Autodesk Inventor part; units mm, degrees
ref_plane "YZ Plane" through (0, 0, 0) normal (1, 0, 0) x (0, 1, 0)
ref_plane "XZ Plane" through (0, 0, 0) normal (0, 1, 0) x (-1, 0, 0)
ref_plane "XY Plane" through (0, 0, 0) normal (0, 0, 1) x (1, 0, 0)
sketch "スケッチ1" plane through (0, 0, 0) normal (0, 0, 1) x (1, 0, 0)
  line L0 (9.4222, 72.3) -> (45.5, 72.3)
  arc A0 (50.5, 67.3) -> (45.5, 72.3) centre (45.5, 67.3) ccw
  line L1 (50.5, 67.3) -> (50.5, 43.9148)
  arc A1 (45.8359, 41.4187) -> (50.5, 43.9148) centre (47.5, 43.9148) ccw
  line L2 (45.8359, 41.4187) -> (7.7581, 66.8038)
  arc A2 (9.4222, 72.3) -> (7.7581, 66.8038) centre (9.4222, 69.3) ccw
  line L3 (31.5778, 32.3) -> (-4.5, 32.3)
  arc A3 (-9.5, 37.3) -> (-4.5, 32.3) centre (-4.5, 37.3) ccw
  line L4 (-9.5, 37.3) -> (-9.5, 60.6852)
  arc A4 (-4.8359, 63.1813) -> (-9.5, 60.6852) centre (-6.5, 60.6852) ccw
  line L5 (-4.8359, 63.1813) -> (33.2419, 37.7962)
  arc A5 (31.5778, 32.3) -> (33.2419, 37.7962) centre (31.5778, 35.3) ccw
  arc A6 (50.5, -32.7) -> (55.5, -27.7) centre (50.5, -27.7) ccw
  line L6 (55.5, -27.7) -> (55.5, 77.3)
  line L7 (55.5, 77.3) -> (-14.5, 77.3)
  line L8 (-14.5, 77.3) -> (-14.5, 27.3)
  line L9 (-14.5, 27.3) -> (-22.2876, 1.4419)
  arc A7 (-16.3774, 4.8724) -> (-22.2876, 1.4419) centre (-17.5, 0) ccw
  arc A8 (-16.3774, 4.8724) -> (-12.2872, 6.71) centre (-15.5442, 8.4886) ccw
  arc A9 (-7.5, 11.8216) -> (-12.2872, 6.71) centre (0, 0) ccw
  line L10 (-7.5, 11.8216) -> (-7.5, 18.5)
  arc A10 (-1.5, 24.5) -> (-7.5, 18.5) centre (-1.5, 18.5) ccw
  line L11 (-1.5, 24.5) -> (42.5, 24.5)
  arc A11 (48.5, 18.5) -> (42.5, 24.5) centre (42.5, 18.5) ccw
  line L12 (48.5, 18.5) -> (48.5, -8.5)
  line L13 (48.5, -8.5) -> (39.5, -8.5)
  arc A12 (31.5, -0.5) -> (39.5, -8.5) centre (39.5, -0.5) ccw
  line L14 (31.5, -0.5) -> (31.5, 8.5)
  line L15 (31.5, 8.5) -> (11.1243, 8.5)
  arc A13 (12.2844, 6.7152) -> (11.1243, 8.5) centre (0, 0) ccw
  arc A14 (12.2844, 6.7152) -> (16.3816, 4.8733) centre (15.5493, 8.5) ccw
  arc A15 (17.5, -5) -> (16.3816, 4.8733) centre (17.5, 0) ccw
  line L16 (17.5, -5) -> (10.0995, -5)
  arc A16 (8.3431, -3.9565) -> (10.0995, -5) centre (10.0995, -3) ccw
  arc A17 (8.3431, -3.9565) -> (-8.3431, -3.9565) centre (0, -8.5) ccw
  arc A18 (-10.0995, -5) -> (-8.3431, -3.9565) centre (-10.0995, -3) ccw
  line L17 (-10.0995, -5) -> (-17.5, -5)
  arc A19 (-22.5, 0) -> (-17.5, -5) centre (-17.5, 0) ccw
  line L18 (-22.5, 0) -> (-22.5, -27.7)
  arc A20 (-22.5, -27.7) -> (-17.5, -32.7) centre (-17.5, -27.7) ccw
  line L19 (-17.5, -32.7) -> (50.5, -32.7)
  circle A21 centre (-17.5, -27.7) radius 1.9
  circle A22 centre (50.5, -27.7) radius 1.9
  line L20 (55.5, -32.7) -> (-22.5, -32.7)
  line L21 (-22.5, -32.7) -> (-22.5, 5)
  line L22 (-22.5, 5) -> (55.5, 5)
  line L23 (55.5, 5) -> (55.5, -32.7)
  arc A23 (-16.3774, 4.8724) -> (-17.5, -5) centre (-17.5, 0) ccw
  point P0 (0, 0)
  point P1 (-17.5, 5)
extrude "押し出し1" add sketch "スケッチ1" along normal blind 3 contours L19 A20 L18 A19 L17 A18 A17 A16 L16 A15 L22 L14 A12 L13 L12 L6 A6 | L12 L13 A12 L14 L22 | A23 A7 A8 L22 A14 A15 L16 A16 A17 A18 L17 A19 | A15 A14 L22 | L22 A8 A7 | A21 | A22
fillet "フィレット1" radius 5 1 edges at (55.5, 5, 1.5)
sketch "スケッチ2" plane through (0, 0, 3) normal (0, 0, 1) x (1, 0, 0)
  circle A0 centre (-17.5, 0) radius 1.4
  circle A1 centre (-17.5, -27.7) radius 1.4
  circle A2 centre (17.5, 0) radius 1.4
  circle A3 centre (40, 0) radius 1.35
  circle A4 centre (50.5, -27.7) radius 1.4
  point P0 (0, 0)
hole "穴1" at (40, 0, 3) at (17.5, 0, 3) at (-17.5, 0, 3) at (-17.5, -27.7, 3) at (50.5, -27.7, 3) direction (0, 0, -1) diameter 3 end through all
properties part number "CaseCover"
Could you check a few things on this model? Use its own coordinates, in mm. Coordinates: 2 decimals unless noted, no trailing zeros. Write each loop counter-clockwise with the first axis right and the second up, starting at its lowest first coordinate (ties: lowest second). Pieces come first, ordered by that corner, then holes. Notation, with made-up numbers: (5.5, 42) - (47.5, 42) arc R25 cw to (47.5, 64) - close; hole circle Ø4 at (9, 40). An arc over 180 degrees is marked (long way). Use a Markdown table: item, result.
Q1. I'm going to push a flat-ended pin straight in: pin 1 Ø2.5 at (x, y) = (40, 0) entering from +Z (3 decimals). Where does the tip first touch, or does it pass through?
Geometry check:
| item | result |
|---|---|
| pin 1 | passes through |
Q2. Imagine slicing it at B-B (z = 2.2). List the corners of the cut face in (x, y) for me, and give its area (3 significant figures).
Geometry check:
| item | result |
|---|---|
| outline | (-22.5, -27.7) arc R5 ccw to (-17.5, -32.7) - (50.5, -32.7) arc R5 ccw to (55.5, -27.7) - (55.5, 0) arc R5 ccw to (50.5, 5) - (-17.5, 5) arc R5 ccw to (-22.29, 1.44) arc R5 ccw to (-22.5, 0) - close; hole circle Ø3 at (-17.5, -27.7); hole circle Ø3 at (-17.5, 0); hole circle Ø3 at (17.5, 0); hole circle Ø3 at (40, 0); hole circle Ø3 at (50.5, -27.7) |
| area | 2,880 mm2 |
Q3. Thinking about a two-plate mould opening in X: for faces 1 (the cylindrical face through (16, 0, 1)), 2 (the flat face through (16, 5, 1)), 3 (the cylindrical face through (-21, -31.27, 1.48)), which applies, +X half, -X half, draft (parallel to the pull), parting line (faces both ways), or undercut?
Geometry check:
| item | result |
|---|---|
| face 1 | undercut |
| face 2 | draft |
| face 3 | -X half |
Q4. Please list where these lines run through material, in increasing order: L1, parallel to Y at x = -17.5, z = 1.4; L2, parallel to X at y = -27.7, z = 2.3; L3, parallel to Y at x = 50.5, z = 1.75.
Geometry check:
| item | result |
|---|---|
| L1 | y = -32.7 to -29.2, -26.2 to -1.5, 1.5 to 5 |
| L2 | x = -22.5 to -19, -16 to 49, 52 to 55.5 |
| L3 | y = -32.7 to -29.2, -26.2 to 5 |
Q5. Imagine slicing it at A-A (x = 17.5). List the corners of the cut face in (y, z) for me.
Geometry check:
| item | result |
|---|---|
| outline | (-32.7, 0) - (-1.5, 0) - (-1.5, 3) - (-32.7, 3) - close; (1.5, 0) - (5, 0) - (5, 3) - (1.5, 3) - close |
